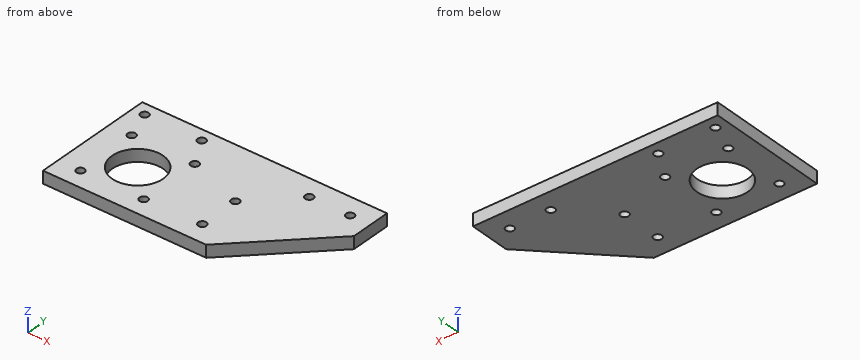
```python
from build123d import *

# Parameters (mm, degrees)
SKETCH1_R           = 2
BOSS_EXTRUDE1_DEPTH = 6
SKETCH2_R           = 2
SKETCH2_R_2         = 12.5
CUT_EXTRUDE1_DEPTH  = 10


with BuildPart() as part:
    # Sketch1 → Boss-Extrude1 (new body)
    with BuildSketch(Plane.XY):
        Polygon((20, -60), (60, -20), (60, 0), (0, 0), (-60, 0), (-60, -60), (0, -60), align=None)
        with Locations((50, -10)):
            Circle(SKETCH1_R, mode=Mode.SUBTRACT)
        with Locations((30, -10)):
            Circle(SKETCH1_R, mode=Mode.SUBTRACT)
        with Locations((10, -50)):
            Circle(SKETCH1_R, mode=Mode.SUBTRACT)
        with Locations((10, -30)):
            Circle(SKETCH1_R, mode=Mode.SUBTRACT)
        with Locations((-54, -6)):
            Circle(SKETCH1_R, mode=Mode.SUBTRACT)
        with Locations((-26, -6)):
            Circle(SKETCH1_R, mode=Mode.SUBTRACT)
    extrude(amount=BOSS_EXTRUDE1_DEPTH)

    # Sketch2 → Cut-Extrude1 (cut)
    with BuildSketch(Plane(origin=(0, 0, 0), x_dir=(-1, 0, 0), z_dir=(0, 0, -1))):
        with Locations((18, -20)):
            Circle(SKETCH2_R)
        with Locations((18, -50.95)):
            Circle(SKETCH2_R)
        with Locations((48.95, -20)):
            Circle(SKETCH2_R)
        with Locations((48.95, -50.95)):
            Circle(SKETCH2_R)
        with Locations((33.475, -35.475)):
            Circle(SKETCH2_R_2)
    extrude(amount=-CUT_EXTRUDE1_DEPTH, mode=Mode.SUBTRACT)


solid = part.part
```
Input: part model. Units: mm. Frame: model coordinates. Coordinates: 2 decimals unless noted, no trailing zeros. Write each loop counter-clockwise with the first axis right and the second up, starting at its lowest first coordinate (ties: lowest second). Pieces come first, ordered by that corner, then holes.
1) Section C-C on x = -48.95. Output: boundary loops of the cut face in (y, z).
2) Section A-A on y = -6. Output: boundary loops of the cut face in (x, z).
3) Material intervals for line 1 along Y through (x, z) = (10, 4.2); line 2 along Y through (x, z) = (-18, 2.6); line 3 along X through (y, z) = (-21.5, 2.05), sorted ascending.
4) Section B-B on x = 50. Output: boundary loops of the cut face in (y, z).
5) Section D-D on z = 1.8. State how many separate pieces and enclosed holes the cut face has, and give its area (3 significant figures).
6) Pin query (flat end, axial travel): pin 1 Ø2.5 at (x, y) = (10, -50) entering from -Z. Return the tip coordinate at first contact, or that it passes through.
Check result:
1. outline: (-60, 0) - (-52.95, 0) - (-52.95, 6) - (-60, 6) - close; (-48.95, 0) - (-22, 0) - (-22, 6) - (-48.95, 6) - close; (-18, 0) - (0, 0) - (0, 6) - (-18, 6) - close
2. outline: (-60, 0) - (-56, 0) - (-56, 6) - (-60, 6) - close; (-52, 0) - (-28, 0) - (-28, 6) - (-52, 6) - close; (-24, 0) - (60, 0) - (60, 6) - (-24, 6) - close
3. line 1: y = -60 to -52, -48 to -32, -28 to 0
3. line 2: y = -60 to -52.95, -48.95 to -22, -18 to 0
3. line 3: x = -60 to -50.27, -47.63 to -19.32, -16.68 to 58.5
4. outline: (-30, 0) - (-12, 0) - (-12, 6) - (-30, 6) - close; (-8, 0) - (0, 0) - (0, 6) - (-8, 6) - close
5. separate pieces: 1
5. enclosed holes: 11
5. area: 5,780 mm2
6. pin 1: passes through
